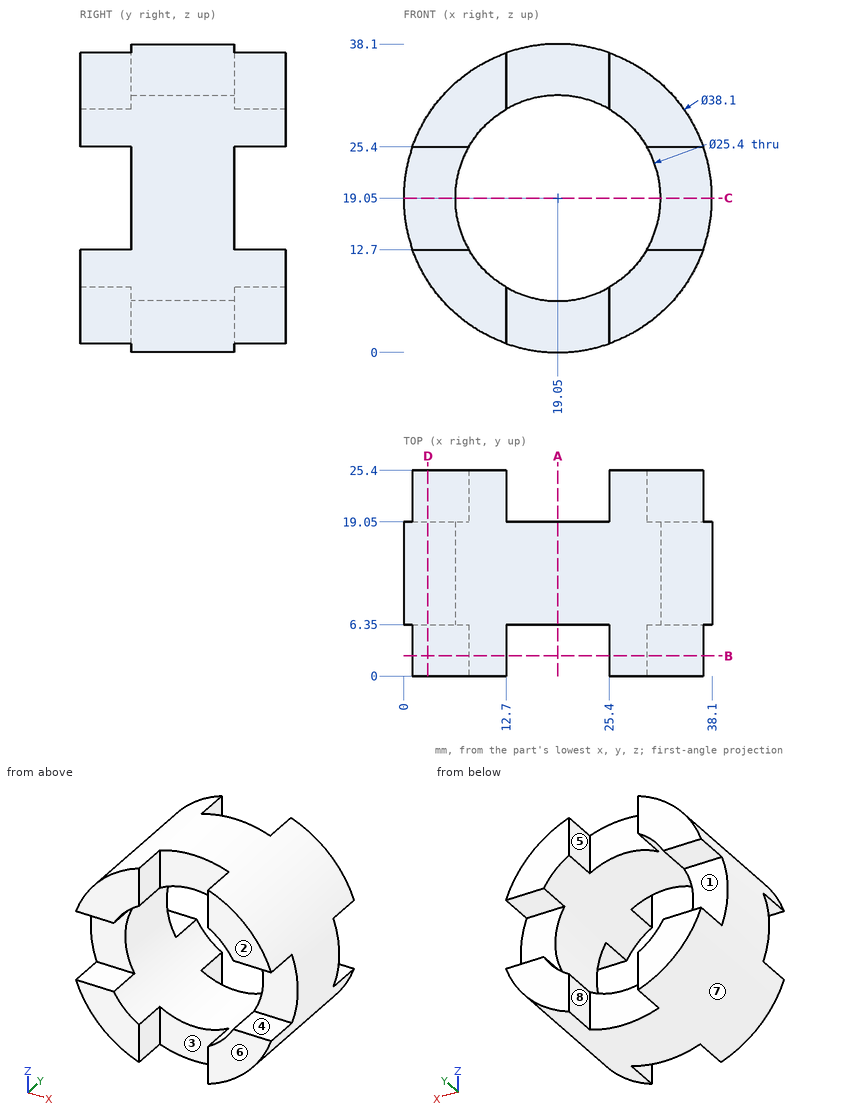
Answer from the drawing. Dimensions are ordinates in mm from the lowest x, y and z of the part. A direction names the side the tool comes from. Round coordinates to 2 decimals unless told otherwise and drop trailing zeros. Write each loop counter-clockwise with the first axis right and the second up, starting at its lowest first coordinate (ties: lowest second). Pieces come first, ordered by that corner, then holes. Notation, with made-up numbers: M -8.75,70.25 L 5.25,70.25 A11 ccw 5.25,77.25 Z; hole C -31,-7.75 d2. An arc over 180 degrees is marked long. Write each question's results on one line, items separated by ' | '. Start each with the question number.
Item 1: For the marked faces 1, 2, 3, 4 and 5, determine the directions among +Z, -Z, +X, -X, +Y, -Y from which every point of the face is accessible in a straight line to the end or side of a thin tool.
Item 2: A cutting plane is placed at D-D on x = 3. Write down the section's boundary in (y, z).
Item 3: A cutting plane is placed at A-A on x = 19.05. Write down the section's boundary in (y, z), and give its area (3 significant figures).
Item 4: Flat-ended cylindrical pins translate along their axes: pin 1 Ø2.5 at (x, z) = (34, 19.5) entering from +Y; pin 2 Ø1.9 at (y, z) = (2.5, 32.5) entering from -X; pin 3 Ø1.9 at (y, z) = (22.5, 4) entering from +X; pin 4 Ø10 at (x, z) = (33.5, 17) entering from -Y. Find the tip coordinate at first contact, or state that the pin passes through.
Item 5: A cutting plane is placed at C-C on z = 19.05. Write down the section's boundary in (x, y), and give its area (3 significant figures).
Item 6: For a pull along X with two mould halves and no side action, classify the marked faces 6, 7 and 8 as pulls with the +X half, pulls with the -X half, needs draft (parallel to the pull), parting line crosses it, or undercut.
Item 7: A cutting plane is placed at B-B on y = 2.5. Write down the section's boundary in (x, z), and give its area (3 significant figures).
Item 8: Straight lines are drawn through the part: L1, parallel to X at y = 6.5, z = 19.05; L2, parallel to X at y = 21, z = 3.5. For each, find the intervals that lie inside material, in ascending order. Write a range as [from, to].
Check sheet entries:
1) face 1: +X, -X, +Y | face 2: +Z, -Z, +X, -X, -Y | face 3: +Z, -Z, -Y | face 4: +X, -X, -Y | face 5: +Z, -Z, +Y
2) outline: M 0,8.79 L 25.4,8.79 L 25.4,12.7 L 19.05,12.7 L 19.05,25.4 L 25.4,25.4 L 25.4,29.31 L 0,29.31 L 0,25.4 L 6.35,25.4 L 6.35,12.7 L 0,12.7 Z
3) outline: M 6.35,0 L 19.05,0 L 19.05,6.35 L 6.35,6.35 Z; M 6.35,31.75 L 19.05,31.75 L 19.05,38.1 L 6.35,38.1 Z | area: 161 mm²
4) pin 1: y = 19.05 | pin 2: x = 4.67 | pin 3: x = 31.86 | pin 4: y = 0
5) outline: M 0,6.35 L 6.35,6.35 L 6.35,19.05 L 0,19.05 Z; M 31.75,6.35 L 38.1,6.35 L 38.1,19.05 L 31.75,19.05 Z | area: 161 mm²
6) face 6: needs draft | face 7: parting line crosses it | face 8: undercut
7) outline: M 1.09,12.7 A19.05 ccw 12.7,1.09 L 12.7,8.05 A12.7 cw 8.05,12.7 Z; M 1.09,25.4 L 8.05,25.4 A12.7 cw 12.7,30.05 L 12.7,37.01 A19.05 ccw Z; M 25.4,1.09 A19.05 ccw 37.01,12.7 L 30.05,12.7 A12.7 cw 25.4,8.05 Z; M 25.4,30.05 A12.7 cw 30.05,25.4 L 37.01,25.4 A19.05 ccw 25.4,37.01 Z | area: 301 mm²
8) L1: [0, 6.35], [31.75, 38.1] | L2: [8.05, 12.7], [25.4, 30.05]
